The listing builds one solid part. Answer for the finished solid, in the listing's coordinates (mm). Round coordinates to 2 decimals unless told otherwise and drop trailing zeros. Use a Markdown table: item, result. Add a question column.
Q1. Given pin 1 Ø8 at (x, y) = (260.5, 9) entering from +Z; pin 2 Ø5 at (x, y) = (143, 8) entering from +Z; pin 3 Ø2 at (x, y) = (202.5, 10.5) entering from +Z, each flat-ended and moving along its own axis, determine where each tip first touches the part or whether it passes through.
Q2. Consider line 1 (X direction, y = 19.5, z = -85.09); line 2 (Z direction, x = 64, y = 15.5); line 3 (Z direction, x = 67.5, y = 16). Determine where each line is inside the solid, lowest interval first.
Q3. Section A-A on y = 18.75 is taken. Give the number of separate pieces and of enclosed holes in the cut face, then the cut area to 3 significant figures.
from build123d import *

# Parameters (mm, degrees)
SKETCH1_R           = 3.175
BOSS_EXTRUDE1_DEPTH = 25.4
FILLET1_R           = 3.175


with BuildPart() as part:
    # Sketch1 (on Top Plane) → Boss-Extrude1 (new body)
    with BuildSketch(Plane(origin=(0, 0, 0), x_dir=(1, 0, 0), z_dir=(0, 1, 0))):
        with BuildLine():
            Line((21.236708827, 102.87), (21.236708827, 0))
            Line((21.236708827, 0), (33.93670901, 0))
            Line((33.93670901, 0), (36.685985199, 0))
            Line((36.685985199, 0), (38.264138871, 3.81))
            Line((38.264138871, 3.81), (51.398278194, 3.81))
            Line((51.398278194, 3.81), (52.996677053, 12.874970388))
            add(Edge.make_bspline(
                [(52.996677053, 12.874970388), (53.503573659, 12.970456896), (54.499660255, 13.157404611), (56.101158607, 13.455975027), (57.663492356, 13.744988885), (59.683937793, 14.115659666), (62.15348224, 14.563331695), (65.170518963, 15.103156387), (68.231004621, 15.644086126), (72.288386319, 16.351836474), (79.324536107, 17.555493521), (89.492362091, 19.238273344), (105.683337087, 21.809296224), (126.007402708, 24.866297862), (158.54183076, 29.467314799), (199.286173571, 34.777983678), (264.569984849, 42.553821851), (346.311852481, 51.162108318), (444.543686218, 60.086524235), (542.885062348, 67.730751053), (624.910991839, 73.034056624), (690.569900499, 76.552162095), (731.621303417, 78.407861838), (764.4690412, 79.64241837), (789.108361632, 80.421082634), (809.63843083, 80.924660048), (826.066348864, 81.194620604), (834.261568503, 81.28), (838.361715067, 81.28)],
                knots=[0.063996746, 0.063996746, 0.063996746, 0.063996746, 0.065824877, 0.067653009, 0.06948114, 0.071309272, 0.074965534, 0.078621797, 0.08227806, 0.085934322, 0.093246848, 0.107871899, 0.122496949, 0.151747051, 0.180997153, 0.239497356, 0.297997559, 0.414997966, 0.531998373, 0.648998779, 0.765999186, 0.824499389, 0.882999593, 0.912249694, 0.941499796, 0.970749898, 0.985374949, 0.999999999, 0.999999999, 0.999999999, 0.999999999], degree=3))
            Line((838.361715067, 81.28), (889.161715067, 81.28))
            Line((889.161715067, 81.28), (916.641442525, 81.28))
            Line((916.641442525, 81.28), (916.641442525, 83.82))
            Line((916.641442525, 83.82), (916.641442525, 102.87))
            Line((916.641442525, 102.87), (21.236708827, 102.87))
        make_face()
        with Locations(Location((859.436708827, 93.345, 0), (0, 0, 90))):
            Circle(SKETCH1_R, mode=Mode.SUBTRACT)
        with Locations(Location((65.686708827, 85.09, 0), (0, 0, 90))):
            Circle(SKETCH1_R, mode=Mode.SUBTRACT)
        with Locations(Location((211.736708827, 61.976, 0), (0, 0, 90))):
            Circle(SKETCH1_R, mode=Mode.SUBTRACT)
        with Locations(Location((630.836708827, 93.345, 0), (0, 0, 90))):
            Circle(SKETCH1_R, mode=Mode.SUBTRACT)
        with Locations(Location((402.236708827, 85.09, 0), (0, 0, 90))):
            Circle(SKETCH1_R, mode=Mode.SUBTRACT)
        with Locations(Location((65.686708827, 35.56, 0), (0, 0, 90))):
            Circle(SKETCH1_R, mode=Mode.SUBTRACT)
    extrude(amount=BOSS_EXTRUDE1_DEPTH)

    # Fillet1
    fillet1_edges = [part.edges().sort_by_distance(p)[0] for p in [
        (52.996677053, 12.7, -12.874970388),
        (38.264138871, 12.7, -3.81),
    ]]
    fillet(fillet1_edges, radius=FILLET1_R)


solid = part.part
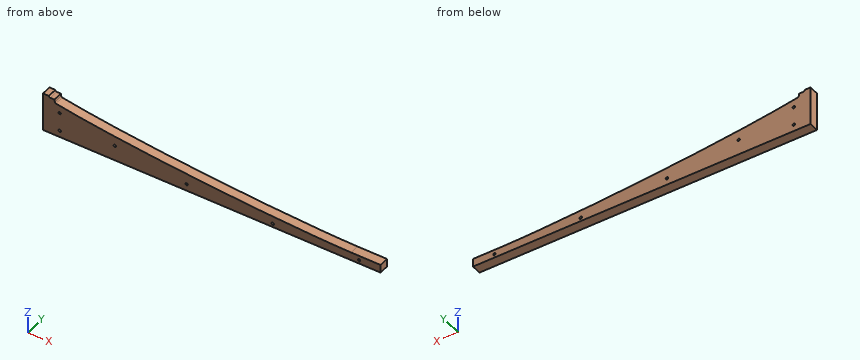
Checked values:
| question | item | result |
|---|---|---|
| 1 | pin 1 | stops at z = -41.47 |
| 1 | pin 2 | stops at z = -26.91 |
| 1 | pin 3 | stops at z = -34.96 |
| 2 | line 1 | x = 21.24 to 62.51, 68.86 to 399.06, 405.41 to 916.64 |
| 2 | line 2 | z = -102.87 to -87.78, -82.4 to -38.25, -32.87 to -14.89 |
| 2 | line 3 | z = -102.87 to -87.7, -82.48 to -38.17, -32.95 to -15.51 |
| 3 | separate pieces | 1 |
| 3 | enclosed holes | 6 |
| 3 | area | 41,400 mm2 |
